Study the drawing (mm; zero at the part's minimum x, y, z) and answer. A direction names the side the tool comes from. Give positions to 0.01 mm unless a question says otherwise; leave off trailing zeros. Write each loop counter-clockwise with the first axis right and the second up, starting at its lowest first coordinate (ties: lowest second). Pieces come first, ordered by that corner, then holes. Notation, with made-up numbers: M 42,-25 L 62,-25 A15 ccw 62,-17 Z; hole C -38.75,-1 d1. An arc over 180 degrees is marked long. Use a Markdown table: item, result. Add a question column.
Item 1: For the marked faces 4 and 5, determine the directions among +Z, -Z, +X, -X, +Y, -Y from which every point of the face is accessible in a straight line to the end or side of a thin tool.
Item 2: Consider probe 1 along Y at (x, z) = (19, 1); probe 2 along Y at (x, z) = (3, 17); probe 3 along X at (y, z) = (36, 27.5). Determine where each line is inside the solid, lowest interval first. Write a range as [from, to].
Item 3: The mould has two halves that part along X. Classify the marked faces 1, 2 and 3: pulls with the +X half, pulls with the -X half, needs draft (parallel to the pull), parting line crosses it, or undercut.
Item 4: A cutting plane is placed at B-B on z = 17. Determine the outline of the cut face in (x, y).
Item 5: Given P1, Ø2, axis at y = 5, z = 17.5, coming from the +X side; P2, Ø1, axis at y = 28.5, z = 26, coming from the +X side; P3, Ø10, axis at y = 23.5, z = 16.5, coming from the -X side, each flat-ended and moving along its own axis, determine where each tip first touches the part or whether it passes through.
Item 6: A cutting plane is placed at C-C on x = 35. Determine the outline of the cut face in (y, z).
Item 7: A cutting plane is placed at D-D on y = 34.5. Count the separate pieces of the cut face and the enclosed holes in it, then the cut area to 3 significant figures.
Item 8: A cutting plane is placed at A-A on y = 6.5. Determine the outline of the cut face in (x, z).
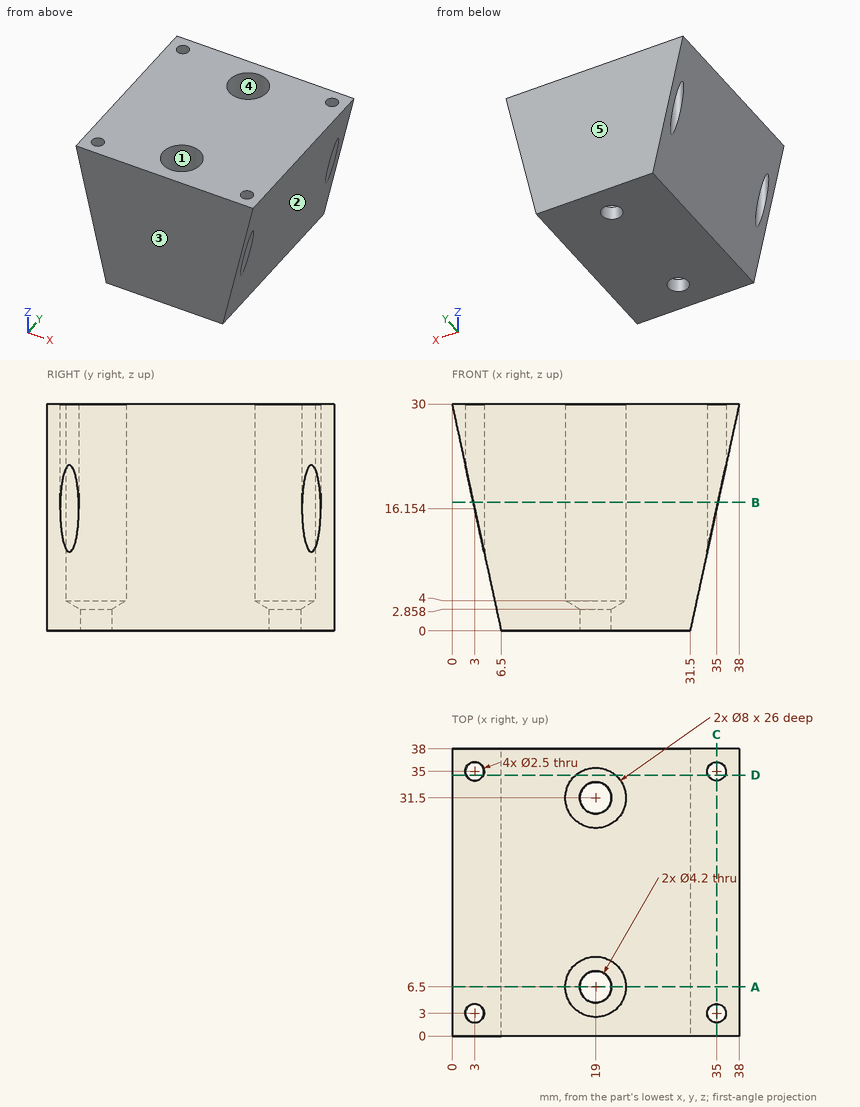
Filled in:
| question | item | result |
|---|---|---|
| 1 | face 4 | +Z |
| 1 | face 5 | +Z, -Z, +X, -X, +Y |
| 2 | probe 1 | [0, 4.4], [8.6, 29.4], [33.6, 38] |
| 2 | probe 2 | [0, 1.75], [4.25, 33.75], [36.25, 38] |
| 2 | probe 3 | [0.54, 2.25], [3.75, 34.25], [35.75, 37.46] |
| 3 | face 1 | undercut |
| 3 | face 2 | pulls with the +X half |
| 3 | face 3 | needs draft |
| 4 | outline | M 2.82,0 L 35.18,0 L 35.18,1.76 A1.25 cw long 35.18,4.24 L 35.18,33.76 A1.25 cw long 35.18,36.24 L 35.18,38 L 2.82,38 L 2.82,36.24 A1.25 cw long 2.82,33.76 L 2.82,4.24 A1.25 cw long 2.82,1.76 Z; hole C 19,6.5 d8; hole C 19,31.5 d8 |
| 5 | P1 | x = 35.51 |
| 5 | P2 | x = 37.24 |
| 5 | P3 | x = 1.84 |
| 6 | outline | M 0,16.15 L 1.75,16.15 L 1.75,30 L 0,30 Z; M 4.25,16.15 L 33.75,16.15 L 33.75,30 L 4.25,30 Z; M 36.25,16.15 L 38,16.15 L 38,30 L 36.25,30 Z |
| 7 | separate pieces | 3 |
| 7 | enclosed holes | 0 |
| 7 | area | 742 mm² |
| 8 | outline | M 0,30 L 6.5,0 L 16.9,0 L 16.9,2.86 L 15,4 L 15,30 Z; M 21.1,0 L 31.5,0 L 38,30 L 23,30 L 23,4 L 21.1,2.86 Z |
